Geometry check sheet. Reference: the model listing, model coordinates, mm. A direction names the side the tool comes from. Coordinates: 2 decimals unless noted, no trailing zeros. Write each loop counter-clockwise with the first axis right and the second up, starting at its lowest first coordinate (ties: lowest second). Pieces come first, ordered by that corner, then holes. Notation, with made-up numbers: (47, -26) -> (54, -26) arc R11 cw to (54, -9) -> close; hole circle Ø11 at (56.5, -29.5). An arc over 180 degrees is marked (long way). One line per question, with ' | ' between items.
```python
from build123d import *

# Parameters (mm, degrees)
F0_R            = 22.225
F0_R_2          = 15.875
F1_DEPTH        = 76.2
F2_R            = 1.5
F3_DEPTH        = 25
F3_COPIES_COUNT = 2
F3_COPIES_ANGLE = 90
F4_R            = 38.1
F4_R_2          = 22.225
F5_DEPTH        = 6.35


# Not quite as in the source:
# - a pattern or mirror of a feature is missing from the dataset's text; its kind, count and spacing are read off the source's solid


with BuildPart() as f1:
    # F0 (on Top) → F1 (new body)
    with BuildSketch(Plane.XY):
        Circle(F0_R)
        Circle(F0_R_2, mode=Mode.SUBTRACT)
    extrude(amount=F1_DEPTH)

    # F2 (on Right) → F3 (cut)
    with BuildSketch(Plane.YZ):
        with Locations((0, 74.041)):
            Circle(F2_R)
    f3 = extrude(amount=-F3_DEPTH, mode=Mode.SUBTRACT)

    # F3_copies: F3 ×2 about axis
    f3_copies_axis = Axis((0, 0, 0), (0, 0, 1))
    for i in range(1, F3_COPIES_COUNT):
        add(f3.rotate(f3_copies_axis, i * F3_COPIES_ANGLE / (F3_COPIES_COUNT - 1)), mode=Mode.SUBTRACT)

    # F4 (on face) → F5 (join)
    with BuildSketch(Plane(origin=(0, 0, 0), x_dir=(1, 0, 0), z_dir=(0, 0, -1))):
        with Locations((0, -0.5167627824)):
            Circle(F4_R)
        Circle(F4_R_2, mode=Mode.SUBTRACT)
    extrude(amount=-F5_DEPTH)


solid = f1.part
```
(1) Draft check along X on faces 4 (the face through (-18.97, 0.69, 72.71)), 5 (the face through (-8.3, 37.7, 3.1)), 6 (the face through (-3.441, -15.497, 37.567)). Enter one of: pulls with the +X half, pulls with the -X half, needs draft (parallel to the pull), parting line crosses it, or undercut.
Answers below:
face 4: needs draft | face 5: parting line crosses it | face 6: undercut
(2) Material ranges on line 1 (X direction, y = 0, z = 36) (3 decimals); line 2 (Z direction, x = 0, y = -18); line 3 (X direction, y = -14.5, z = 39.5), recorded low to high.
Answers below:
line 1: x = -22.225 to -15.875, 15.875 to 22.225 | line 2: z = 0 to 72.54, 75.54 to 76.2 | line 3: x = -16.84 to -6.46, 6.46 to 16.84
(3) Cross-section at D-D (y = 19). Record the cut outline in (x, z).
Answers below:
outline: (-33.32, 0) -> (33.32, 0) -> (33.32, 6.35) -> (11.53, 6.35) -> (11.53, 76.2) -> (-11.53, 76.2) -> (-11.53, 6.35) -> (-33.32, 6.35) -> close
(4) Tool access check on faces 1 (the face through (21.199, 6.676, 40.786)), 2 (the face through (-0.69, -18.97, 72.71)), 3 (the face through (10, -15, 76.2)). Record the directions out of +Z, -Z, +X, -X, +Y, -Y that give a thin tool (end or side, any length) a straight path to the whole face; none if there is none.
Answers below:
face 1: +Z | face 2: -Y | face 3: +Z, +X, -X, +Y, -Y
(5) Cross-section at A-A (x = 0). Record the cut outline in (y, z) (3 decimals), plus the area to 3 significant figures.
Answers below:
outline: (-37.583, 0) -> (-15.875, 0) -> (-15.875, 72.541) -> (-22.225, 72.541) -> (-22.225, 6.35) -> (-37.583, 6.35) -> close; (-22.225, 75.541) -> (-15.875, 75.541) -> (-15.875, 76.2) -> (-22.225, 76.2) -> close; (15.875, 0) -> (38.617, 0) -> (38.617, 6.35) -> (22.225, 6.35) -> (22.225, 76.2) -> (15.875, 76.2) -> close | area: 1,150 mm²
(6) Depth check by flat-ended pin: P1, Ø3, axis at x = -2.5, z = 17.5, coming from the +Y side; P2, Ø10, axis at x = 16.5, z = 13.5, coming from the +Y side; P3, Ø4, axis at y = 0, z = 74.041, coming from the -X side (3 decimals). Enter the tip coordinate at first touch or a pass-through.
Answers below:
P1: stops at y = 22.2 | P2: stops at y = 19.02 | P3: stops at x = -22.225
(7) Cross-section at B-B (y = -13). Record the cut outline in (x, z), plus the area to 3 significant figures.
Answers below:
outline: (-35.62, 0) -> (-9.11, 0) -> (-9.11, 76.2) -> (-18.03, 76.2) -> (-18.03, 6.35) -> (-35.62, 6.35) -> close; (9.11, 0) -> (35.62, 0) -> (35.62, 6.35) -> (18.03, 6.35) -> (18.03, 76.2) -> (9.11, 76.2) -> close | area: 1,580 mm²
(8) Cross-section at C-C (z = 9.5). Record the cut outline in (x, y) (3 decimals), plus the area to 3 significant figures.
Answers below:
outline: circle Ø44.45 at (0, 0); hole circle Ø31.75 at (0, 0) | area: 760 mm²
